The figure shows three views and two pictorial views of one solid part (mm, origin at its lowest corner). Answer the questions. Coordinates: 2 decimals unless noted, no trailing zeros. Write each loop counter-clockwise with the first axis right and the second up, starting at its lowest first coordinate (ties: lowest second). Pieces come first, ordered by that corner, then holes. Notation, with made-up numbers: M 78.25,-15 L 128.25,-15 A37 ccw 128.25,22 Z; hole C 16,-20.75 d8. An arc over 180 degrees is marked long. Write item = value, one per line.
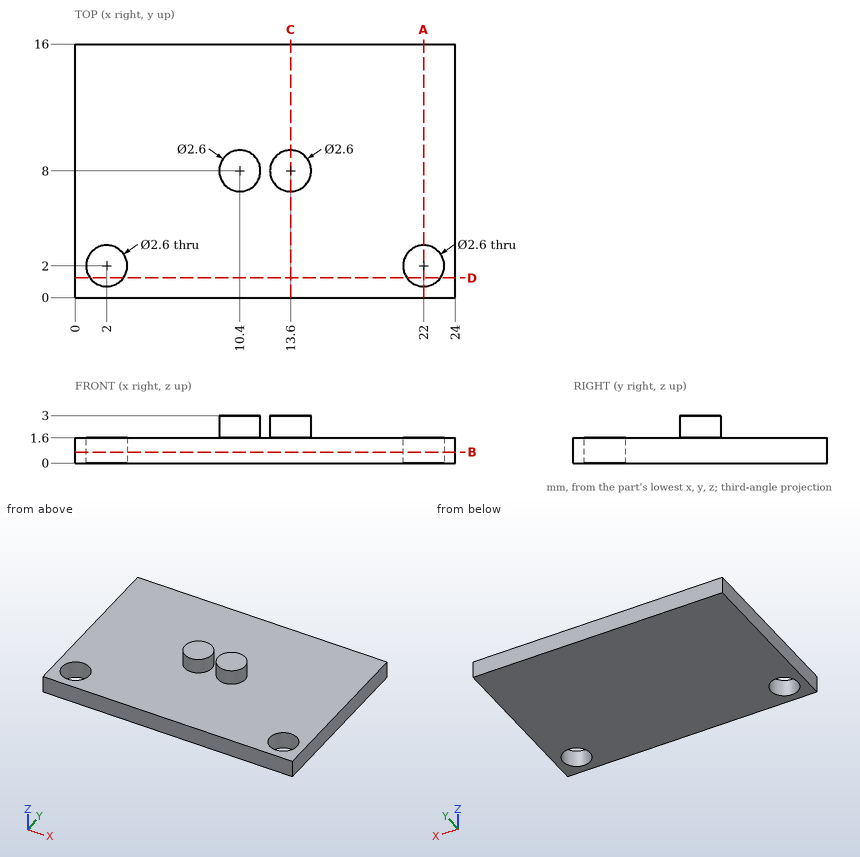
Item 1: Consider line 1 along X through (y, z) = (2, 0.6); line 2 along Y through (x, z) = (2, 0.65); line 3 along Y through (x, z) = (10.5, 1.8). Determine where each line is inside the solid, lowest interval first. Write a range as from..to.
Worked answers:
line_1 = 0..0.7, 3.3..20.7, 23.3..24
line_2 = 0..0.7, 3.3..16
line_3 = 6.7..9.3
Item 2: Find section B-B (z = 0.7). Determine the outline of the cut face in (x, y).
Worked answers:
outline = M 0,0 L 24,0 L 24,16 L 0,16 Z; hole C 2,2 d2.6; hole C 22,2 d2.6
Item 3: Find section A-A (x = 22). Determine the outline of the cut face in (y, z).
Worked answers:
outline = M 0,0 L 0.7,0 L 0.7,1.6 L 0,1.6 Z; M 3.3,0 L 16,0 L 16,1.6 L 3.3,1.6 Z
Item 4: Find section D-D (y = 1.25). Determine the outline of the cut face in (x, z).
Worked answers:
outline = M 0,0 L 0.94,0 L 0.94,1.6 L 0,1.6 Z; M 3.06,0 L 20.94,0 L 20.94,1.6 L 3.06,1.6 Z; M 23.06,0 L 24,0 L 24,1.6 L 23.06,1.6 Z
Item 5: Find section C-C (x = 13.6). Determine the outline of the cut face in (y, z).
Worked answers:
outline = M 0,0 L 16,0 L 16,1.6 L 9.3,1.6 L 9.3,3 L 6.7,3 L 6.7,1.6 L 0,1.6 Z
Item 6: A flat-ended cylindrical pin translates along its axis: pin 1 (3.5 mm diameter, centred on x = 22, y = 2, fed in from +Z). Find the tip coordinate at first contact, or state that the pin passes through.
Worked answers:
pin_1 = 1.6
